from build123d import *

# Parameters (mm, degrees)
BOSS_EXTRUDE1_DEPTH                          = 34
FILLET1_R                                    = 1
SKETCH2_R                                    = 1.5
CUT_EXTRUDE3_DEPTH                           = 10
CSK_FOR_M1_6_COUNTERSUNK_FLAT_HEAD_S_2_COUNT = 2
CSK_FOR_M1_6_COUNTERSUNK_FLAT_HEAD_S_2_PITCH = 8
LPATTERN1_COUNT                              = 2
LPATTERN1_PITCH                              = 10
LPATTERN2_COUNT                              = 2
LPATTERN2_PITCH                              = 10


with BuildPart() as part:
    # Sketch1 → Boss-Extrude1 (new body)
    with BuildSketch(Plane(origin=(0, 0, 0), x_dir=(0, 0, -1), z_dir=(1, 0, 0))):
        Polygon((0, 15), (0, 0), (15, 0), (15, 2), (2, 2), (2, 15), align=None)
    extrude(amount=BOSS_EXTRUDE1_DEPTH)

    # Fillet1
    fillet1_edges = [part.edges().sort_by_distance(p)[0] for p in [
        (17, 2, -2),
    ]]
    fillet(fillet1_edges, radius=FILLET1_R)

    # Sketch2 → Cut-Extrude3 (cut)
    with BuildSketch(Plane.XZ):
        with Locations(Location((28.999999992, -7.999999993, 0), (0, 0, 270))):
            Circle(SKETCH2_R)
        with Locations(Location((5, -8, 0), (0, 0, 270))):
            Circle(SKETCH2_R)
    extrude(amount=-CUT_EXTRUDE3_DEPTH, mode=Mode.SUBTRACT)

    # Sketch4 → CSK for M1.6 Countersunk Flat Head Screw1 (revolve, cut)
    with BuildSketch(Plane(origin=(17, 5, -2), x_dir=(0, 1, 0), z_dir=(1, 0, 0))):
        Polygon((0, 0), (0, 30.540774557), (0.9, 30), (0.9, 0.9), (1.8, 0), align=None)
    csk_for_m1_6_countersunk_flat_head_screw = revolve(axis=Axis((17, 5, -8.35), (0, 0, 1)), mode=Mode.SUBTRACT)

    # CSK for M1.6 Countersunk Flat Head S 2: CSK for M1.6 Countersunk Flat Head Screw1 ×2
    with Locations(*[(0, i * CSK_FOR_M1_6_COUNTERSUNK_FLAT_HEAD_S_2_PITCH, 0) for i in range(1, CSK_FOR_M1_6_COUNTERSUNK_FLAT_HEAD_S_2_COUNT)]):
        add(csk_for_m1_6_countersunk_flat_head_screw, mode=Mode.SUBTRACT)

    # LPattern1: CSK for M1.6 Countersunk Flat Head Screw1 ×2
    with Locations(*[(-i * LPATTERN1_PITCH, 0, 0) for i in range(1, LPATTERN1_COUNT)]):
        add(csk_for_m1_6_countersunk_flat_head_screw, mode=Mode.SUBTRACT)

    # LPattern1 copy 1 sketch → LPattern1 copy 1 (revolve, cut)
    with BuildSketch(Plane(origin=(7, 13, -2), x_dir=(0, 1, 0), z_dir=(1, 0, 0))):
        Polygon((0, 0), (0, 30.540774557), (0.9, 30), (0.9, 0.9), (1.8, 0), align=None)
    revolve(axis=Axis((7, 13, -8.35), (0, 0, 1)), mode=Mode.SUBTRACT)

    # LPattern2: CSK for M1.6 Countersunk Flat Head Screw1 ×2
    with Locations(*[(i * LPATTERN2_PITCH, 0, 0) for i in range(1, LPATTERN2_COUNT)]):
        add(csk_for_m1_6_countersunk_flat_head_screw, mode=Mode.SUBTRACT)

    # LPattern2 copy 1 sketch → LPattern2 copy 1 (revolve, cut)
    with BuildSketch(Plane(origin=(27, 13, -2), x_dir=(0, 1, 0), z_dir=(1, 0, 0))):
        Polygon((0, 0), (0, 30.540774557), (0.9, 30), (0.9, 0.9), (1.8, 0), align=None)
    revolve(axis=Axis((27, 13, -8.35), (0, 0, 1)), mode=Mode.SUBTRACT)


solid = part.part
Here's how the part is built. I have some questions about the finished solid (model axes, mm). A direction names the side the tool comes from. Coordinates: 2 decimals unless noted, no trailing zeros. Order: outer loops, then holes, each group sorted by start corner. A loop starts at its lowest first (then second) coordinate and runs counter-clockwise, first axis right, second up. Notation, with made-up numbers: M 17.5,46.5 L 44.5,46.5 A22 cw 44.5,66.5 Z; hole C 74.25,30 d5. An arc over 180 degrees is marked long. Answer as CSV lines item,"result".
Item 1: We'd pull the mould along X, two halves only. Please class faces 3 (the face through (0, 5, -1)), 4 (the face through (5.07, 0.99, -6.5)), 5 (the face through (17, 0, -7)): +X half, -X half, draft (parallel to the pull), parting line (faces both ways), or undercut.
Results found:
face 3,"-X half"
face 4,"undercut"
face 5,"draft"
Item 2: Imagine slicing it at B-B on z = -8. Write out the boundary of the cut face in (x, y).
Results found:
outline,"M 0,0 L 3.5,0 L 3.5,2 L 0,2 Z; M 6.5,0 L 27.5,0 L 27.5,2 L 6.5,2 Z; M 30.5,0 L 34,0 L 34,2 L 30.5,2 Z"
Item 3: On a 3-axis mill with a long thin cutter (end or side, diameter ignored), from which of +Z, -Z, +X, -X, +Y, -Y can I reach the whole of each face in a straight line? I mean faces 1 (the face through (17, 9, -2)), 2 (the face through (7, 4.1, -0.6)). Say none if no direction works.
Results found:
face 1,"-Z, +X, -X, +Y"
face 2,"+Z, -Z"
Item 4: If I drill on line 1 (Y direction, x = 27, z = -0.8); line 2 (X direction, y = 13, z = -0.8); line 3 (X direction, y = 0.6, z = -8), over which ranges is the centre line in solid material (lowest first)?
Results found:
line 1,"0 to 4.1, 5.9 to 12.1, 13.9 to 15"
line 2,"0 to 6.1, 7.9 to 16.1, 17.9 to 26.1, 27.9 to 34"
line 3,"0 to 3.5, 6.5 to 27.5, 30.5 to 34"
Item 5: Imagine slicing it at C-C on y = 5. Write out the boundary of the cut face in (x, z).
Results found:
outline,"M 0,-2 L 5.2,-2 L 6.1,-1.1 L 6.1,0 L 0,0 Z; M 7.9,-1.1 L 8.8,-2 L 15.2,-2 L 16.1,-1.1 L 16.1,0 L 7.9,0 Z; M 17.9,-1.1 L 18.8,-2 L 25.2,-2 L 26.1,-1.1 L 26.1,0 L 17.9,0 Z; M 27.9,-1.1 L 28.8,-2 L 34,-2 L 34,0 L 27.9,0 Z"
Item 6: For pin 1 (3 mm diameter, centred on x = 27, y = 13, fed in from -Z); pin 2 (2 mm diameter, centred on x = 18, y = 13, fed in from -Z); pin 3 (2 mm diameter, centred on x = 17, y = 13, fed in from -Z), each with a flat end and sliding along its axis, tell me the tip position at first contact or that it passes through.
Results found:
pin 1,"z = -1.7"
pin 2,"z = -2"
pin 3,"z = -1.2"
Item 7: Imagine slicing it at A-A on x = 17. Write out the boundary of the cut face in (y, z), plus the area to 3 significant figures.
Results found:
outline,"M 0,-15 L 2,-15 L 2,-3 A1 cw 3,-2 L 3.2,-2 L 4.1,-1.1 L 4.1,0 L 0,0 Z; M 5.9,-1.1 L 6.8,-2 L 11.2,-2 L 12.1,-1.1 L 12.1,0 L 5.9,0 Z; M 13.9,-1.1 L 14.8,-2 L 15,-2 L 15,0 L 13.9,0 Z"
area,"47.4 mm2"
Item 8: Imagine slicing it at D-D on y = 10.5. Write out the boundary of the cut face in (x, z), plus the area to 3 significant figures.
Results found:
outline,"M 0,-2 L 34,-2 L 34,0 L 0,0 Z"
area,"68.0 mm2"
